Geometry: final body of the model. Coordinates: model frame, mm. Give positions to 0.01 mm unless a question says otherwise; leave off trailing zeros. Write each loop counter-clockwise with the first axis right and the second up, starting at its lowest first coordinate (ties: lowest second). Pieces come first, ordered by that corner, then holes. Notation, with made-up numbers: (57.25, -33.75) -> (98.25, -33.75) arc R24 ccw to (98.25, -7.75) -> close; hole circle Ø9 at (-26, 6). An arc over 180 degrees is marked (long way). Answer in a Markdown table with one row per item. Add a question column.
from build123d import *

# Parameters (mm, degrees)
F0_R     = 39.3
F0_R_2   = 38.5
F1_DEPTH = 1.2
F2_DEPTH = 50
F4_SIZE  = 0.5


# Not quite as in the source:
# - a fillet or chamfer that OpenCascade refuses, or shapes differently, is made with other operations: its cross-section is extruded or revolved along the edge and cut away or added


with BuildPart() as f1:
    # F0 (on Top) → F1 (new body)
    with BuildSketch(Plane.XY):
        Circle(F0_R)
        Circle(F0_R_2, mode=Mode.SUBTRACT)
        Circle(F0_R_2)
    extrude(amount=-F1_DEPTH)

    # F0 (on Top) → F2 (join)
    with BuildSketch(Plane.XY):
        Circle(F0_R)
        Circle(F0_R_2, mode=Mode.SUBTRACT)
    extrude(amount=F2_DEPTH)

    # F3: chamfer of 1 on 1 edges, made by hand

    # F3_s1 → F3_t2 (revolve, cut)
    with BuildSketch(Plane.XZ):
        Polygon((39.5, 50), (38.5, 49), (38.5, 50), align=None)
    revolve(axis=Axis((0, 0, 50), (0, 0, 1)), mode=Mode.SUBTRACT)

    # F4
    f4_edges = [f1.edges().sort_by_distance(p)[0] for p in [
        (-39.3, 0, -1.2),
    ]]
    chamfer(f4_edges, length=F4_SIZE)


solid = f1.part
Q1. Line query: probe 1 along Y at (x, z) = (0, 19.5); probe 2 along Z at (x, y) = (-11, -14); probe 3 along Y at (x, z) = (-29, 42). Output: solid intervals per line, ascending. Write a range as from..to.
Q2. Contact query for flat-ended pins moving along their axis: pin 1 Ø1 at (x, z) = (-12, 27) entering from -Y; pin 2 Ø1 at (x, z) = (2, 5) entering from -Y; pin 3 Ø5 at (x, y) = (-3, 4.5) entering from +Z. Output: stop coordinate, or through.
Q3. Section C-C on z = 7. Return loops of the section in (x, y), and give its area (3 significant figures).
Q4. Pull-direction query (Y, two-part tool) for faces 1 (the flat face through (-1, 1, 0)), 2 (the conical face through (36, -15, -1)), 3 (the flat face through (-1, 1, -1.2)); classes: +Y half, -Y half, draft (parallel to the pull), parting line (faces both ways), or undercut.
Q5. Section A-A on y = 0. Return loops of the section in (x, z).
Checks:
| question | item | result |
|---|---|---|
| 1 | probe 1 | -39.3..-38.5, 38.5..39.3 |
| 1 | probe 2 | -1.2..0 |
| 1 | probe 3 | -26.52..-25.32, 25.32..26.52 |
| 2 | pin 1 | y = -37.58 |
| 2 | pin 2 | y = -39.27 |
| 2 | pin 3 | z = 0 |
| 3 | outline | circle Ø78.6 at (0, 0); hole circle Ø77 at (0, 0) |
| 3 | area | 196 mm^2 |
| 4 | face 1 | undercut |
| 4 | face 2 | parting line |
| 4 | face 3 | draft |
| 5 | outline | (-39.3, -0.7) -> (-38.8, -1.2) -> (38.8, -1.2) -> (39.3, -0.7) -> (39.3, 49.8) -> (38.5, 49) -> (38.5, 0) -> (-38.5, 0) -> (-38.5, 49) -> (-39.3, 49.8) -> close |
